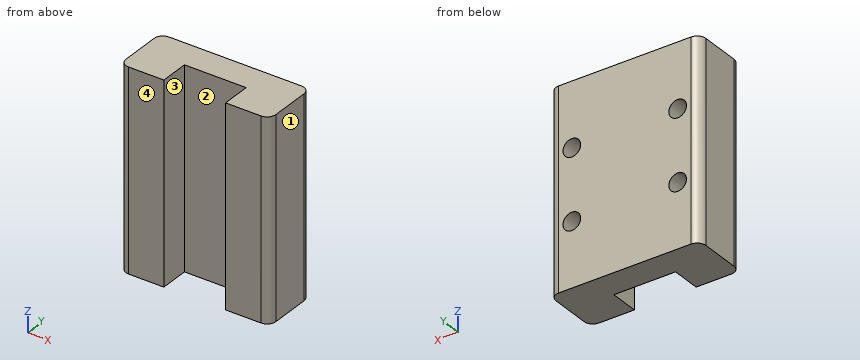
```python
from build123d import *

# Parameters (mm, degrees)
EXTRUDE_1_DEPTH     = 22.5
SKETCH_2_R          = 1
CUT_EXTRUDE_1_DEPTH = 2.5


with BuildPart() as part:
    # 草图1 → 凸台-拉伸1 (new body)
    with BuildSketch(Plane.XY):
        with BuildLine():
            Line((5, 3.3), (12, 3.3))
            Line((12, 3.3), (12, 0))
            Line((12, 0), (16, 0))
            ThreePointArc((16, 0), (16.707106781, 0.292893219), (17, 1))
            Line((17, 1), (17, 5.5))
            ThreePointArc((17, 5.5), (16.707106781, 6.207106781), (16, 6.5))
            Line((16, 6.5), (1, 6.5))
            ThreePointArc((1, 6.5), (0.292893219, 6.207106781), (0, 5.5))
            Line((0, 5.5), (0, 1))
            ThreePointArc((0, 1), (0.292893219, 0.292893219), (1, 0))
            Line((1, 0), (5, 0))
            Line((5, 0), (5, 3.3))
        make_face()
    extrude(amount=EXTRUDE_1_DEPTH)

    # 草图2 → 切除-拉伸1 (cut)
    with BuildSketch(Plane(origin=(0, 6.5, 0), x_dir=(1, 0, 0), z_dir=(0, 1, 0))):
        with Locations((2.5, -15.25)):
            Circle(SKETCH_2_R)
        with Locations((2.5, -7.25)):
            Circle(SKETCH_2_R)
        with Locations((14.5, -7.25)):
            Circle(SKETCH_2_R)
        with Locations((14.5, -15.25)):
            Circle(SKETCH_2_R)
    extrude(amount=-CUT_EXTRUDE_1_DEPTH, mode=Mode.SUBTRACT)


solid = part.part
```
The listing builds one solid part. Answer for the finished solid, in the listing's coordinates (mm). Face numbers are marked on the shaded views. Give positions to 0.01 mm unless a question says otherwise; leave off trailing zeros. Loops run counter-clockwise (first coordinate to the right, second up) from the corner with the lowest first, then second, coordinate; pieces in that order, holes last. Notation, with made-up numbers: (84.5, -17.75) - (106.5, -17.75) arc R19 ccw to (106.5, 10.25) - close; hole circle Ø4 at (36.25, 27.5). An arc over 180 degrees is marked (long way). Answer as CSV lines item,"result". Start each with the question number.
Item 1: Find the intervals of material crossed by line 1 (X direction, y = 5.45, z = 15.25); line 2 (Z direction, x = 2.5, y = 4.65); line 3 (X direction, y = 3.25, z = 7.25), in increasing order. Write a range as from..to.
Item 2: A cutting plane is placed at A-A on y = 3. Determine the outline of the cut face in (x, z), then the cut area to 3 significant figures.
Item 3: A cutting plane is placed at C-C on x = 2.5. Determine the outline of the cut face in (y, z).
Item 4: The mould has two halves that part along X. Classify the marked faces 1, 2, 3 and 4: +X half, -X half, draft (parallel to the pull), parting line (faces both ways), or undercut.
Item 5: A cutting plane is placed at B-B on z = 10.75. Determine the outline of the cut face in (x, y).
Item 6: A cutting plane is placed at D-D on z = 7.25. Determine the outline of the cut face in (x, y), then the cut area to 3 significant figures.
Item 7: Each of these flat-tipped pins is pushed along its axis until it touches: pin 1 (0.6 mm diameter, centred on x = 14.5, z = 15, fed in from +Y); pin 2 (1.6 mm diameter, centred on x = 14, z = 7.5, fed in from +Y); pin 3 (5.5 mm diameter, centred on x = 8.5, z = 12.5, fed in from -Y). Where does it stop, or does it pass through?
Found:
1,line 1,"x = 0..1.5, 3.5..13.5, 15.5..17"
1,line 2,"z = 0..6.25, 8.25..14.25, 16.25..22.5"
1,line 3,"x = 0..5, 12..17"
2,outline,"(0, 0) - (5, 0) - (5, 22.5) - (0, 22.5) - close; (12, 0) - (17, 0) - (17, 22.5) - (12, 22.5) - close"
2,area,"225 mm^2"
3,outline,"(0, 0) - (6.5, 0) - (6.5, 6.25) - (4, 6.25) - (4, 8.25) - (6.5, 8.25) - (6.5, 14.25) - (4, 14.25) - (4, 16.25) - (6.5, 16.25) - (6.5, 22.5) - (0, 22.5) - close"
4,face 1,"+X half"
4,face 2,"undercut"
4,face 3,"undercut"
4,face 4,"draft"
5,outline,"(0, 1) arc R1 ccw to (1, 0) - (5, 0) - (5, 3.3) - (12, 3.3) - (12, 0) - (16, 0) arc R1 ccw to (17, 1) - (17, 5.5) arc R1 ccw to (16, 6.5) - (1, 6.5) arc R1 ccw to (0, 5.5) - close"
6,outline,"(0, 1) arc R1 ccw to (1, 0) - (5, 0) - (5, 3.3) - (12, 3.3) - (12, 0) - (16, 0) arc R1 ccw to (17, 1) - (17, 5.5) arc R1 ccw to (16, 6.5) - (15.5, 6.5) - (15.5, 4) - (13.5, 4) - (13.5, 6.5) - (3.5, 6.5) - (3.5, 4) - (1.5, 4) - (1.5, 6.5) - (1, 6.5) arc R1 ccw to (0, 5.5) - close"
6,area,"76.5 mm^2"
7,pin 1,"stops at y = 4"
7,pin 2,"stops at y = 6.5"
7,pin 3,"stops at y = 3.3"
